from build123d import *


with BuildPart() as part:
    # Sketch1 → Revolve-Thin1 (revolve)
    with BuildSketch(Plane(origin=(0, 0, 0), x_dir=(0, 0, -1), z_dir=(1, 0, 0)), mode=Mode.PRIVATE) as revolve_thin1_sk:
        Polygon((0, 16), (-3, 16), (-5.2, 18.2), (-5.2, 38), (-3, 38), (-3, 38.4), (-5.6, 38.4), (-5.6, 18.034314575), (-3.165685425, 15.6), (0, 15.6), align=None)
    revolve(revolve_thin1_sk.sketch.rotate(Axis((0, 0, 0), (0, 0, 1)), 90), axis=Axis((0, 0, 0), (0, 0, 1)))


solid = part.part
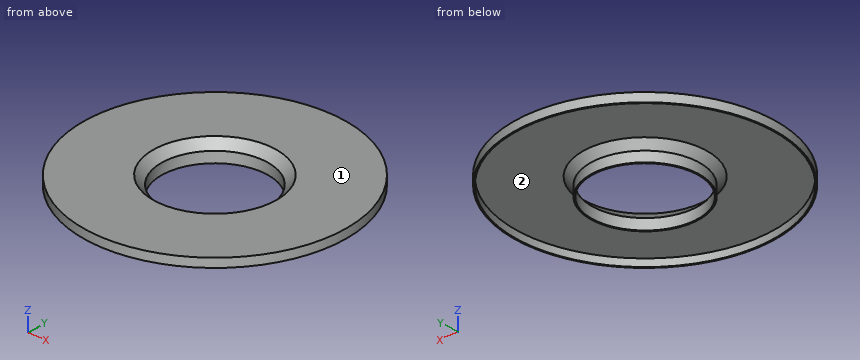
Source: CAD feature listing. Evaluate the final solid. Frame: model axes, mm. Face numbers are marked on the shaded views. Give positions to 0.01 mm unless a question says otherwise; leave off trailing zeros. Loops run counter-clockwise (first coordinate to the right, second up) from the corner with the lowest first, then second, coordinate; pieces in that order, holes last. Notation, with made-up numbers: (-25, -2) -> (30, -2) arc R18 cw to (30, 20) -> close; hole circle Ø2 at (-14.75, 57.5). An arc over 180 degrees is marked (long way). Use a Markdown table: item, result. Add a question column.
1) Pull-direction query (X, two-part tool) for the marked faces 1 and 2; classes: +X half, -X half, draft (parallel to the pull), parting line (faces both ways), or undercut.
2) Section query A-A, the plane x = 0. Return the cut outline in (y, z).
3) Section query D-D, the plane y = -26. Return the cut outline in (x, z).
4) Section query C-C, the plane z = 1.4. Return the cut outline in (x, y), then the cut area to 3 significant figures.
5) First-contact query: pin 1 (25 mm diameter, centred on x = 0, y = 0, fed in from -Z); pin 2 (5 mm diameter, centred on x = 17, y = -2, fed in from +Z); pin 3 (12 mm diameter, centred on x = 27, y = -19, fed in from -Z); pin 4 (3 mm diameter, centred on x = 13, z = 4.5, fed in from +Y). Flat tips, straight axial feed; report the tip coordinate or a pass-through.
6) Line query: line 1 along Y through (x, z) = (0, 0.75); line 2 along Y through (x, z) = (0, 3.55); line 3 along Y through (x, z) = (0, 3.9). Output: solid intervals per line, ascending. Write a range as [from, to].
Numbers:
| question | item | result |
|---|---|---|
| 1 | face 1 | draft |
| 1 | face 2 | undercut |
| 2 | outline | (-38.4, 3) -> (-38, 3) -> (-38, 5.2) -> (-18.2, 5.2) -> (-16, 3) -> (-16, 0) -> (-15.6, 0) -> (-15.6, 3.17) -> (-18.03, 5.6) -> (-38.4, 5.6) -> close; (15.6, 0) -> (16, 0) -> (16, 3) -> (18.2, 5.2) -> (38, 5.2) -> (38, 3) -> (38.4, 3) -> (38.4, 5.6) -> (18.03, 5.6) -> (15.6, 3.17) -> close |
| 3 | outline | (-28.26, 3) -> (-27.71, 3) -> (-27.71, 5.2) -> (27.71, 5.2) -> (27.71, 3) -> (28.26, 3) -> (28.26, 5.6) -> (-28.26, 5.6) -> close |
| 4 | outline | circle Ø32 at (0, 0); hole circle Ø31.2 at (0, 0) |
| 4 | area | 39.7 mm2 |
| 5 | pin 1 | passes through |
| 5 | pin 2 | stops at z = 5.6 |
| 5 | pin 3 | stops at z = 3 |
| 5 | pin 4 | stops at y = 36.64 |
| 6 | line 1 | y = [-16, -15.6], [15.6, 16] |
| 6 | line 2 | y = [-38.4, -38], [-16.55, -15.98], [15.98, 16.55], [38, 38.4] |
| 6 | line 3 | y = [-38.4, -38], [-16.9, -16.33], [16.33, 16.9], [38, 38.4] |
